```python
from build123d import *

# Parameters (mm, degrees)
SKETCH2_W           = 104.14
SKETCH2_H           = 69.85
BOSS_EXTRUDE1_DEPTH = 11.43
SKETCH3_W           = 71.12
SKETCH3_H           = 28.179594488
CUT_EXTRUDE1_DEPTH  = 9.652
CUT_EXTRUDE2_DEPTH  = 7.62
SKETCH5_R           = 2.032
CUT_EXTRUDE3_DEPTH  = 12.7
FILLET1_R           = 6.35


with BuildPart() as part:
    # Sketch2 → Boss-Extrude1 (new body)
    with BuildSketch(Plane(origin=(0, 0, 0), x_dir=(1, 0, 0), z_dir=(0, 1, 0))):
        Rectangle(SKETCH2_W, SKETCH2_H)
    extrude(amount=BOSS_EXTRUDE1_DEPTH)

    # Sketch3 → Cut-Extrude1 (cut)
    with BuildSketch(Plane(origin=(0, 11.43, 0), x_dir=(1, 0, 0), z_dir=(0, 1, 0))):
        with Locations((-6.35, 23.614797244)):
            Rectangle(SKETCH3_W, SKETCH3_H)
    extrude(amount=-CUT_EXTRUDE1_DEPTH, mode=Mode.SUBTRACT)

    # Sketch4 → Cut-Extrude2 (cut)
    with BuildSketch(Plane(origin=(0, 11.43, 0), x_dir=(1, 0, 0), z_dir=(0, 1, 0))):
        Polygon((49.149, 30.226), (-49.149, 30.226), (-49.149, -30.226), (-49.149, -30.48), (49.149, -30.48), (49.149, -30.226), align=None)
    extrude(amount=-CUT_EXTRUDE2_DEPTH, mode=Mode.SUBTRACT)

    # Sketch5 → Cut-Extrude3 (cut)
    with BuildSketch(Plane(origin=(0, 11.43, 0), x_dir=(1, 0, 0), z_dir=(0, 1, 0))):
        with Locations(Location((-46.609, 27.84475, 0), (0, 0, 270))):
            Circle(SKETCH5_R)
        with Locations(Location((46.609, 27.84475, 0), (0, 0, 270))):
            Circle(SKETCH5_R)
        with Locations(Location((46.609, -27.84475, 0), (0, 0, 270))):
            Circle(SKETCH5_R)
        with Locations(Location((-46.609, -27.84475, 0), (0, 0, 270))):
            Circle(SKETCH5_R)
    extrude(amount=-CUT_EXTRUDE3_DEPTH, mode=Mode.SUBTRACT)

    # Fillet1
    fillet1_edges = [part.edges().sort_by_distance(p)[0] for p in [
        (-52.07, 5.715, -34.925),
        (52.07, 5.715, -34.925),
        (52.07, 5.715, 34.925),
        (-52.07, 5.715, 34.925),
    ]]
    fillet(fillet1_edges, radius=FILLET1_R)


solid = part.part
```
Here's how the part is built. I have some questions about the finished solid (model axes, mm). A direction names the side the tool comes from. Give positions to 0.01 mm unless a question says otherwise; leave off trailing zeros. Loops run counter-clockwise (first coordinate to the right, second up) from the corner with the lowest first, then second, coordinate; pieces in that order, holes last. Notation, with made-up numbers: M 89.25,23.25 L 110.25,23.25 A16 cw 110.25,44.25 Z; hole C 66,-25 d11. An arc over 180 degrees is marked long. Put each result on its own line as item: value. Start each with the question number.
(1) I want a section at C-C on z = -5. Please give me the cut outline in (x, y).
(2) If we mould it in two halves opening along Z, with no side actions, what happens to faces 4 (the flat face through (-41.91, 3, -28)), 5 (the flat face through (-1, 6, 34.925)), 6 (the cylindrical face through (-44.594, 1.932, 27.58))? For each: +Z half, -Z half, draft (parallel to the pull), parting line (faces both ways), or undercut.
(3) I want a section at A-A on x = 43.5. Please give me the cut outline in (y, z) (3 decimals), then the cut area to 3 significant figures.
(4) I need wall thicknesses on line 1 along X through (y, z) = (8.5, -15); line 2 along Z through (x, y) = (-46, 2); line 3 along Z through (x, y) = (40, 7.5) (3 decimals). Which ranges of each line are inside material? Lowest first, please. Write a range as [from, to].
(5) I want a section at D-D on z = -22.5. Please give me the cut outline in (x, y), then the cut area to 3 significant figures.
(6) Will these pins go through, and if not, where does the flat tip stop? pin 1 Ø3.5 at (x, y) = (-47, 8.5) entering from +Z (3 decimals); pin 2 Ø0.6 at (x, y) = (-14.5, 2.5) entering from -Z (3 decimals); pin 3 Ø2 at (x, y) = (-23.5, 9.5) entering from -Z; pin 4 Ø12.5 at (x, z) = (-6.5, -19.5) entering from +Y.
(7) I want a section at B-B on y = 5. Please give me the cut outline in (x, z) (3 decimals), then the cut area to 3 significant figures.
(8) For faces 1 (the flat face through (-7, 1.778, -22)), 2 (the flat face through (0, 11.43, 31)), 3 (the flat face through (49.149, 8, 1)), which set-ups out of +Z, -Z, +X, -X, +Y, -Y let a thin tool reach every point of the face, with its end or its side?
Answer block:
1. outline: M -52.07,0 L 52.07,0 L 52.07,11.43 L 49.15,11.43 L 49.15,3.81 L -49.15,3.81 L -49.15,11.43 L -52.07,11.43 Z
2. face 4: draft
2. face 5: +Z half
2. face 6: undercut
3. outline: M 0,-34.925 L 11.43,-34.925 L 11.43,-30.226 L 3.81,-30.226 L 3.81,30.48 L 11.43,30.48 L 11.43,34.925 L 0,34.925 Z
3. area: 336 mm^2
4. line 1: [-52.07, -49.15], [49.15, 52.07]
4. line 2: [-34.92, -29.78], [-25.91, 25.91], [29.78, 34.92]
4. line 3: [-34.925, -30.226], [30.48, 34.925]
5. outline: M -52.07,0 L 52.07,0 L 52.07,11.43 L 49.15,11.43 L 49.15,3.81 L 29.21,3.81 L 29.21,1.78 L -41.91,1.78 L -41.91,3.81 L -49.15,3.81 L -49.15,11.43 L -52.07,11.43 Z
5. area: 297 mm^2
6. pin 1: z = 34.925
6. pin 2: z = -9.525
6. pin 3: z = 30.48
6. pin 4: y = 1.78
7. outline: M -52.07,-28.575 A6.35 ccw -45.72,-34.925 L -41.91,-34.925 L -41.91,-30.226 L -49.149,-30.226 L -49.149,30.48 L 49.149,30.48 L 49.149,-30.226 L 29.21,-30.226 L 29.21,-34.925 L 45.72,-34.925 A6.35 ccw 52.07,-28.575 L 52.07,28.575 A6.35 ccw 45.72,34.925 L -45.72,34.925 A6.35 ccw -52.07,28.575 Z
7. area: 938 mm^2
8. face 1: -Z, +Y
8. face 2: +Z, -Z, +X, -X, +Y
8. face 3: +Y
